Read the model definition and answer for the solid it produces. Units are mm, in the model's axes. A direction names the side the tool comes from. Coordinates: 2 decimals unless noted, no trailing zeros. Loops run counter-clockwise (first coordinate to the right, second up) from the corner with the lowest first, then second, coordinate; pieces in that order, holes last.
from build123d import *

# Parameters (mm, degrees)
SKETCH1_R           = 10
BOSS_EXTRUDE1_DEPTH = 30


with BuildPart() as part:
    # Sketch1 → Boss-Extrude1 (new body)
    with BuildSketch(Plane.XY):
        with BuildLine():
            Line((-38.125206472, -20.755714087), (41.874793528, -20.755714087))
            Line((41.874793528, -20.755714087), (41.874793528, -25.755714087))
            Line((41.874793528, -25.755714087), (51.874793528, -25.755714087))
            Line((51.874793528, -25.755714087), (51.874793528, -15.755714087))
            Line((51.874793528, -15.755714087), (21.874793528, -15.755714087))
            Line((21.874793528, -15.755714087), (21.874793528, 4.244285913))
            ThreePointArc((21.874793528, 4.244285913), (1.874793528, 24.244285913), (-18.125206472, 4.244285913))
            Line((-18.125206472, 4.244285913), (-18.125206472, -15.755714087))
            Line((-18.125206472, -15.755714087), (-48.125206472, -15.755714087))
            Line((-48.125206472, -15.755714087), (-48.125206472, -25.755714087))
            Line((-48.125206472, -25.755714087), (-38.125206472, -25.755714087))
            Line((-38.125206472, -25.755714087), (-38.125206472, -20.755714087))
        make_face()
        with Locations((1.874793528, 4.244285913)):
            Circle(SKETCH1_R, mode=Mode.SUBTRACT)
    extrude(amount=BOSS_EXTRUDE1_DEPTH)


solid = part.part
Item 1: A cutting plane is placed at B-B on z = 12.75. Determine the outline of the cut face in (x, y), then the cut area to 3 significant figures.
Numbers:
outline: (-48.13, -25.76) - (-38.13, -25.76) - (-38.13, -20.76) - (41.87, -20.76) - (41.87, -25.76) - (51.87, -25.76) - (51.87, -15.76) - (21.87, -15.76) - (21.87, 4.24) arc R20 ccw to (-18.13, 4.24) - (-18.13, -15.76) - (-48.13, -15.76) - close; hole circle Ø20 at (1.87, 4.24)
area: 1,710 mm2
Item 2: Which of the six approach directions +Z, -Z, +X, -X, +Y, -Y give full straight-line access (tool end or side, diameter ignored) to faces 5 (the face through (37, -15.756, 15)), 6 (the face through (47, -25.756, 15)), 7 (the face through (41.875, -23, 15))?
Numbers:
face 5: +Z, -Z, +X, +Y
face 6: +Z, -Z, +X, -X, -Y
face 7: +Z, -Z, -Y
Item 3: Find the intervals of material crossed by line 1 along X through (y, z) = (-9, 2.5); line 2 along Y through (x, z) = (32, 2.25); line 3 along X through (y, z) = (0.5, 17.75), in increasing order.
Numbers:
line 1: x = -18.13 to 21.87
line 2: y = -20.76 to -15.76
line 3: x = -18.13 to -7.4, 11.15 to 21.87
Item 4: Determine the mould class of faces 1 (the face through (21.875, -6, 15)), 2 (the face through (-18.125, -6, 15)), 3 (the face through (1, -20.756, 15)), 4 (the face through (-33, -15.756, 15)) for opening direction X: released by +X, released by -X, zero draft, split by the parting line, or undercut.
Numbers:
face 1: released by +X
face 2: released by -X
face 3: undercut
face 4: zero draft
Item 5: A cutting plane is placed at C-C on y = -3.5. Determine the outline of the cut face in (x, z), then the cut area to 3 significant figures.
Numbers:
outline: (-18.13, 0) - (-4.45, 0) - (-4.45, 30) - (-18.13, 30) - close; (8.2, 0) - (21.87, 0) - (21.87, 30) - (8.2, 30) - close
area: 820 mm2
Item 6: Given pin 1 (15 mm diameter, centred on x = 42, z = 16, fed in from +Y); pin 2 (6 mm diameter, centred on y = -10.5, z = 20, fed in from +X); pin 3 (10 mm diameter, centred on x = 14, z = 24.5, fed in from -Y); pin 4 (5 mm diameter, centred on x = -6.5, y = 16.5, fed in from -Z), each flat-ended and moving along its own axis, determine where each tip first touches the part or whether it passes through.
Numbers:
pin 1: stops at y = -15.76
pin 2: stops at x = 21.87
pin 3: stops at y = -20.76
pin 4: stops at z = 0
Item 7: A cutting plane is placed at A-A on y = 5.5. Determine the outline of the cut face in (x, z), then the cut area to 3 significant figures.
Numbers:
outline: (-18.09, 0) - (-8.05, 0) - (-8.05, 30) - (-18.09, 30) - close; (11.8, 0) - (21.84, 0) - (21.84, 30) - (11.8, 30) - close
area: 602 mm2
Item 8: A cutting plane is placed at D-D on x = 32.5. Determine the outline of the cut face in (y, z).
Numbers:
outline: (-20.76, 0) - (-15.76, 0) - (-15.76, 30) - (-20.76, 30) - close
